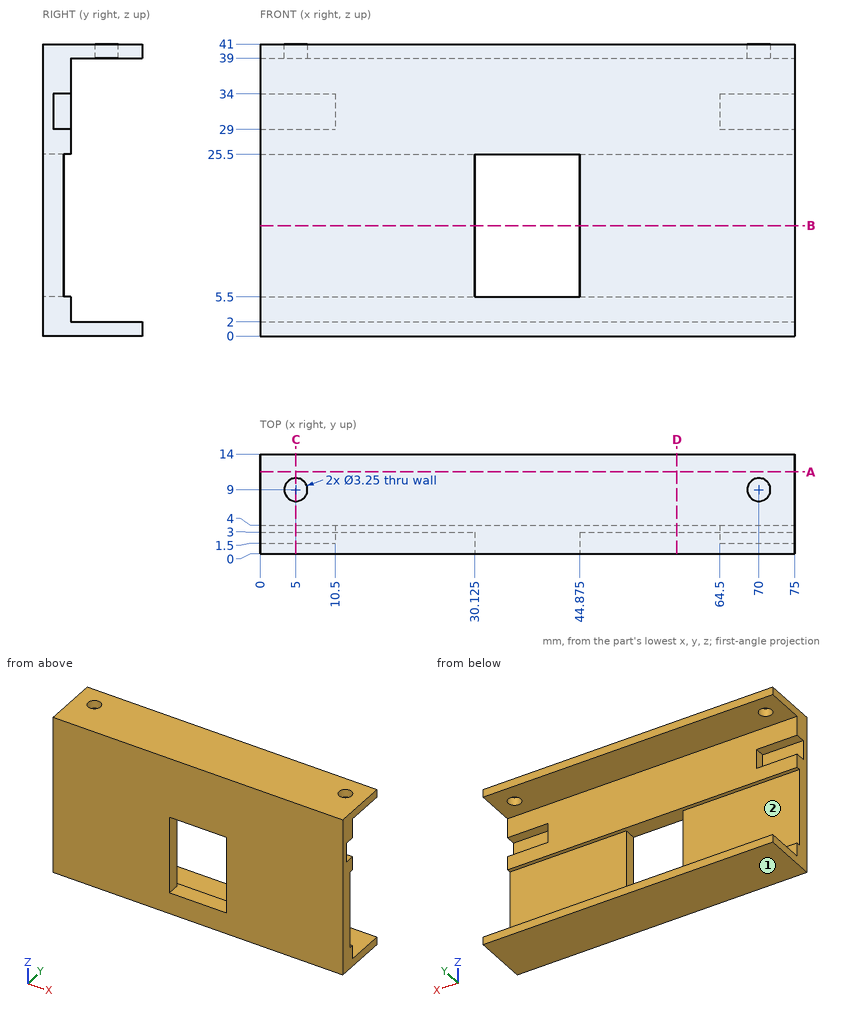
Design review of the part shown in the three views and the two pictorial views. Dimensions are in mm from the part's minimum x, y and z. A direction names the side the tool comes from. Round coordinates to 2 decimals unless told otherwise and drop trailing zeros. Write each loop counter-clockwise with the first axis right and the second up, starting at its lowest first coordinate (ties: lowest second). Pieces come first, ordered by that corner, then holes.
Item 1: We need section C-C on x = 5. Write out the cut boundary in (y, z) (3 decimals).
Item 2: For probe 1 along Z at (x, y) = (17.5, 5.5); probe 2 along Y at (x, z) = (70, 40.25) (3 decimals); probe 3 along Z at (x, y) = (69.5, 2), list the stretches that pass through material, from the lowest coordinate up.
Item 3: We need section B-B on z = 15.5. Write out the cut boundary in (x, y) (3 decimals).
Item 4: We need section A-A on y = 11.5. Write out the cut boundary in (x, z), and give its area (3 significant figures).
Item 5: Clearance check with flat-ended pins moving along their axes: pin 1 Ø1.9 at (x, y) = (5, 9) entering from -Z; pin 2 Ø11 at (x, z) = (19.5, 32.5) entering from +Y; pin 3 Ø2.5 at (x, z) = (3.5, 31.5) entering from +Y; pin 4 Ø3 at (x, z) = (57.5, 9.5) entering from +Y. State where each tip first meets the part, or that it passes through.
Item 6: For the marked faces 1 and 2, list the 3-axis set-ups (+Z, -Z, +X, -X, +Y, -Y) from which the entire face can be reached by the end or side of a thin tool; tool diameter is ignored.
Item 7: We need section D-D on x = 58.5. Write out the cut boundary in (y, z), and give its area (3 significant figures).
Returned:
1. outline: (0, 0) - (14, 0) - (14, 2) - (4, 2) - (4, 5.5) - (3, 5.5) - (3, 25.5) - (4, 25.5) - (4, 29) - (1.5, 29) - (1.5, 34) - (4, 34) - (4, 39) - (7.375, 39) - (7.375, 41) - (0, 41) - close; (10.625, 39) - (14, 39) - (14, 41) - (10.625, 41) - close
2. probe 1: z = 0 to 2, 39 to 41
2. probe 2: y = 0 to 7.375, 10.625 to 14
2. probe 3: z = 0 to 29, 34 to 41
3. outline: (0, 0) - (30.125, 0) - (30.125, 3) - (0, 3) - close; (44.875, 0) - (75, 0) - (75, 3) - (44.875, 3) - close
4. outline: (0, 0) - (75, 0) - (75, 2) - (0, 2) - close; (0, 39) - (75, 39) - (75, 41) - (0, 41) - close
4. area: 300 mm2
5. pin 1: stops at z = 0
5. pin 2: stops at y = 4
5. pin 3: stops at y = 1.5
5. pin 4: stops at y = 3
6. face 1: -Z, +X, -X, +Y, -Y
6. face 2: +X, -X, +Y
7. outline: (0, 0) - (14, 0) - (14, 2) - (4, 2) - (4, 5.5) - (3, 5.5) - (3, 25.5) - (4, 25.5) - (4, 39) - (14, 39) - (14, 41) - (0, 41) - close
7. area: 184 mm2
